from build123d import *

# Parameters (mm, degrees)
SKETCH1_R           = 3
BOSS_EXTRUDE1_DEPTH = 6
BOSS_EXTRUDE2_DEPTH = 3
SKETCH3_R           = 7.85
CUT_EXTRUDE1_DEPTH  = 1
SKETCH4_R           = 6.75
CUT_EXTRUDE2_DEPTH  = 5.2
SKETCH5_W           = 10.298947731
SKETCH5_H           = 6.677630872
BOSS_EXTRUDE3_DEPTH = 0.8
SKETCH6_R           = 3
CUT_EXTRUDE3_DEPTH  = 0.8
BOSS_EXTRUDE5_START = -6
SKETCH7_R           = 9.071835919
SKETCH7_R_2         = 3
SKETCH7_R_3         = 8.53010645
BOSS_EXTRUDE5_DEPTH = 6
SKETCH8_R           = 7.85
CUT_EXTRUDE4_DEPTH  = 1
SKETCH9_R           = 6.75
CUT_EXTRUDE5_DEPTH  = 5.2
BOSS_EXTRUDE6_DEPTH = 3
CUT_EXTRUDE10_DEPTH = 3


with BuildPart() as part:
    # Sketch1 → Boss-Extrude1 (new body)
    with BuildSketch(Plane.XY):
        Polygon((4.142135624, 10), (-4.142135624, 10), (-11.642135624, 2.5), (-96.276080567, 2.5), (-110.474741511, -6.507268438), (-120.82549793, -4.191703376), (-127.82091412, -8.629417024), (-129.629482932, -16.713860663), (-125.191769284, -23.709276854), (-117.107325644, -25.517845665), (-110.111909454, -21.080132017), (-107.796344392, -10.729375598), (-94.823919433, -2.5), (-11.642135624, -2.5), (-4.142135624, -10), (4.142135624, -10), (10, -4.142135624), (10, 4.142135624), align=None)
        with Locations((-118.966411787, -14.85477452)):
            Circle(SKETCH1_R, mode=Mode.SUBTRACT)
        with Locations((-0.876614201, 0)):
            Circle(SKETCH1_R, mode=Mode.SUBTRACT)
    extrude(amount=-BOSS_EXTRUDE1_DEPTH)

    # Sketch2 → Boss-Extrude2 (add)
    with BuildSketch(Plane.XY):
        Polygon((-113.924993651, -5.735413417), (-110.474741511, -6.507268438), (-96.276080567, 2.5), (-11.642135624, 2.5), (-9.142135624, 5), (-97.002161134, 5), align=None)
        Polygon((-108.568199413, -14.179627738), (-107.796344392, -10.729375598), (-94.823919433, -2.5), (-11.642135624, -2.5), (-9.142135624, -5), (-94.097838866, -5), align=None)
    extrude(amount=-BOSS_EXTRUDE2_DEPTH)

    # Sketch3 → Cut-Extrude1 (cut)
    with BuildSketch(Plane(origin=(0, 0, -6), x_dir=(-1, 0, 0), z_dir=(0, 0, -1))):
        Circle(SKETCH3_R)
        with Locations((118.966411787, -14.85477452)):
            Circle(SKETCH3_R)
    extrude(amount=-CUT_EXTRUDE1_DEPTH, mode=Mode.SUBTRACT)

    # Sketch4 → Cut-Extrude2 (cut)
    with BuildSketch(Plane(origin=(0, 0, -6), x_dir=(-1, 0, 0), z_dir=(0, 0, -1))):
        Circle(SKETCH4_R)
        with Locations((118.966411787, -14.85477452)):
            Circle(SKETCH4_R)
    extrude(amount=-CUT_EXTRUDE2_DEPTH, mode=Mode.SUBTRACT)

    # Sketch5 → Boss-Extrude3 (add)
    with BuildSketch(Plane.XY):
        with Locations((-0.876614202, 0)):
            Rectangle(SKETCH5_W, SKETCH5_H)
    extrude(amount=-BOSS_EXTRUDE3_DEPTH)

    # Sketch6 → Cut-Extrude3 (cut)
    with BuildSketch(Plane.XY):
        Circle(SKETCH6_R)
    extrude(amount=-CUT_EXTRUDE3_DEPTH, mode=Mode.SUBTRACT)

    # Sketch7 → Boss-Extrude5 (add)
    # profile 1 of 2: a face of its own
    with BuildSketch(Plane(origin=(0, 0, -6), x_dir=(-1, 0, 0), z_dir=(0, 0, -1)).offset(BOSS_EXTRUDE5_START)):
        Circle(SKETCH7_R)
        with Locations(Location((0, 0, 0), (0, 0, 180))):
            Circle(SKETCH7_R_2, mode=Mode.SUBTRACT)
    # profile 2 of 2: a face of its own
    with BuildSketch(Plane(origin=(0, 0, -6), x_dir=(-1, 0, 0), z_dir=(0, 0, -1)).offset(BOSS_EXTRUDE5_START)):
        with Locations((118.966411787, -14.85477452)):
            Circle(SKETCH7_R_3)
        with Locations(Location((118.966411787, -14.85477452, 0), (0, 0, 180))):
            Circle(SKETCH7_R_2, mode=Mode.SUBTRACT)
    extrude(amount=BOSS_EXTRUDE5_DEPTH)

    # Sketch8 → Cut-Extrude4 (cut)
    with BuildSketch(Plane.XY):
        with Locations((-118.966411787, -14.85477452)):
            Circle(SKETCH8_R)
        Circle(SKETCH8_R)
    extrude(amount=-CUT_EXTRUDE4_DEPTH, mode=Mode.SUBTRACT)

    # Sketch9 → Cut-Extrude5 (cut)
    with BuildSketch(Plane.XY):
        with Locations((-118.966411787, -14.85477452)):
            Circle(SKETCH9_R)
        Circle(SKETCH9_R)
    extrude(amount=-CUT_EXTRUDE5_DEPTH, mode=Mode.SUBTRACT)

    # Sketch10 → Boss-Extrude6 (add)
    with BuildSketch(Plane(origin=(0, 0, -3), x_dir=(-1, 0, 0), z_dir=(0, 0, -1))):
        Polygon((9.142135624, -5), (11.642135624, -2.5), (94.823919433, -2.5), (107.796344392, -10.729375598), (108.568199413, -14.179627738), (94.097838866, -5), align=None)
        Polygon((9.142135624, 5), (11.642135624, 2.5), (96.276080567, 2.5), (110.474741511, -6.507268438), (113.924993651, -5.735413417), (97.002161134, 5), align=None)
    extrude(amount=BOSS_EXTRUDE6_DEPTH)

    # Sketch11 → Cut-Extrude10 (cut)
    with BuildSketch(Plane.XY):
        Polygon((-9.142135624, 5), (-97.002161134, 5), (-113.924993651, -5.735413417), (-110.474741511, -6.507268438), (-96.276080567, 2.5), (-11.642135624, 2.5), align=None)
        Polygon((-11.642135624, -2.5), (-94.823919433, -2.5), (-107.796344392, -10.729375598), (-108.568199413, -14.179627738), (-94.097838866, -5), (-9.142135624, -5), align=None)
    extrude(amount=-CUT_EXTRUDE10_DEPTH, mode=Mode.SUBTRACT)


solid = part.part
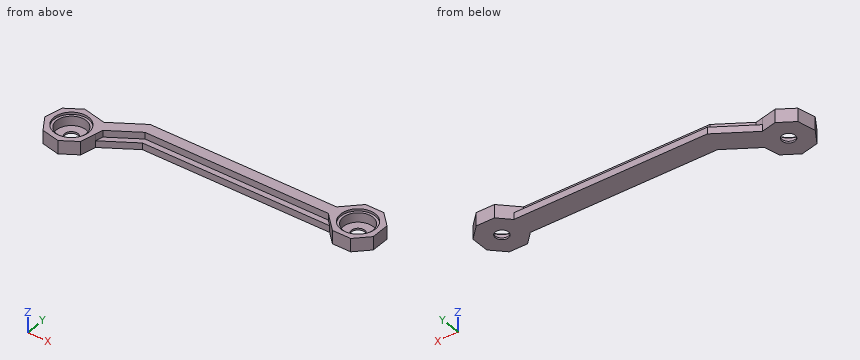
Part model, mm, in its own coordinate system. Round coordinates to 2 decimals unless told otherwise and drop trailing zeros. Loops run counter-clockwise (first coordinate to the right, second up) from the corner with the lowest first, then second, coordinate; pieces in that order, holes last. Notation, with made-up numbers: (-3, 27.5) - (11, 27.5) arc R8 cw to (11, 41.5) - close; hole circle Ø3 at (-28, 72.25). An arc over 180 degrees is marked (long way). Answer as a JSON object with one key per item and string values.
Item 1: Pin check, flat tips, straight feed: pin 1 (2 mm diameter, centred on x = -33.5, z = -1, fed in from -Y); pin 2 (3 mm diameter, centred on x = -7.5, y = -10, fed in from -Z); pin 3 (8 mm diameter, centred on x = 0, y = 0, fed in from +Z); pin 4 (1.5 mm diameter, centred on x = -70, z = -5, fed in from -Y). Stop position of each tip, or through.
Output:
{"pin 1": "y = -2.5", "pin 2": "through", "pin 3": "z = -5.2", "pin 4": "y = -5"}
Item 2: Band-saw the part on B-B on y = 0. List the corners of the cut face in (x, z).
Output:
{"outline": "(-104.88, -6) - (-3, -6) - (-3, -5.2) - (-6.75, -5.2) - (-6.75, -1) - (-7.85, -1) - (-7.85, 0) - (-100.22, 0) - (-100.22, -3) - (-104.88, -3) - close; (3, -6) - (10, -6) - (10, 0) - (7.85, 0) - (7.85, -1) - (6.75, -1) - (6.75, -5.2) - (3, -5.2) - close"}
Item 3: Wall check: L1, parallel to Y at x = 0, z = -5.55; L2, parallel to X at y = -3, z = -2.55; L3, parallel to Z at x = -67.5, y = 4.5. Give the ranges that are in metal, low to high.
Output:
{"L1": "-10 to -3, 3 to 10", "L2": "-104.95 to -95.61, -11.14 to -6.05, 6.05 to 10", "L3": "-6 to -3"}
Item 4: Band-saw the part on C-C on x = -41. List the corners of the cut face in (y, z).
Output:
{"outline": "(-5, -6) - (5, -6) - (5, -3) - (2.5, -3) - (2.5, 0) - (-2.5, 0) - (-2.5, -3) - (-5, -3) - close"}
Item 5: Band-saw the part on A-A on x = 0. List the corners of the cut face in (y, z), plus the area to 3 significant figures.
Output:
{"outline": "(-10, -6) - (-3, -6) - (-3, -5.2) - (-6.75, -5.2) - (-6.75, -1) - (-7.85, -1) - (-7.85, 0) - (-10, 0) - close; (3, -6) - (10, -6) - (10, 0) - (7.85, 0) - (7.85, -1) - (6.75, -1) - (6.75, -5.2) - (3, -5.2) - close", "area": "42.8 mm2"}
